from build123d import *

# Parameters (mm, degrees)
F0_R     = 33.1615614797
F1_DEPTH = 79.248
F3_DEPTH = 111.252
F4_T     = -2.54


with BuildPart() as f1:
    # F0 (on Front) → F1 (new body)
    with BuildSketch(Plane.XZ):
        Circle(F0_R)
    extrude(amount=F1_DEPTH)

    # F2 (on face) → F3 (cut)
    with BuildSketch(Plane.XZ.offset(79.248)):
        Polygon((-9.8989819324, -13.7179617404), (5.2176722472, -3.2694421143), (-0.0481573892, 14.3361204783), (-18.4192732631, 14.7684369255), (-24.507417648, -2.5699394088), align=None)
    extrude(amount=-F3_DEPTH, mode=Mode.SUBTRACT)

    # F4
    f4_openings = [f1.faces().sort_by_distance(p)[0] for p in [
        (-32.223611, -79.248, 0),
    ]]
    offset(amount=F4_T, openings=f4_openings, kind=Kind.INTERSECTION)


solid = f1.part
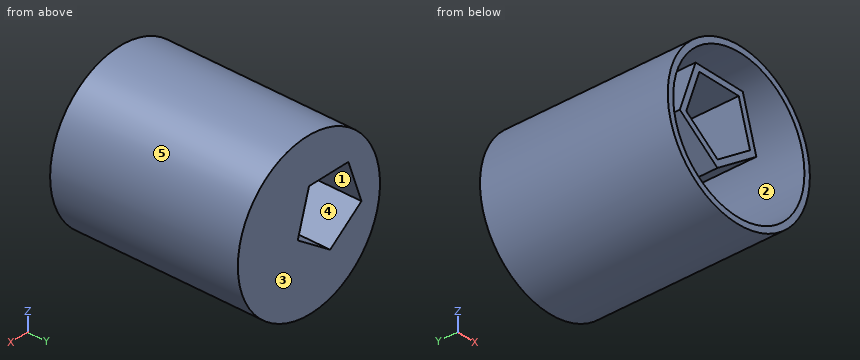
Check sheet for the modelled part. Datum: model origin and axes. Units: mm. Face numbers are marked on the shaded views. A direction names the side the tool comes from. Round coordinates to 2 decimals unless told otherwise and drop trailing zeros. Order: outer loops, then holes, each group sorted by start corner. A loop starts at its lowest first (then second) coordinate and runs counter-clockwise, first axis right, second up.
Q1. Scan lines: L1, parallel to X at y = -51, z = 13; L2, parallel to X at y = -29, z = -6; L3, parallel to Z at x = -2.5, y = -23. Record each from-to range of solid material in increasing order.
Filled sheet:
L1: x = -30.51 to -27.73, -21.73 to -19.04, 0.35 to 3, 27.73 to 30.51
L2: x = -32.61 to -30.03, -24.2 to -20.01, 1.27 to 5.73, 30.03 to 32.61
L3: z = -33.07 to -30.52, -11.69 to -8.6, 14.39 to 16.93, 30.52 to 33.07
Q2. Set-up check for the marked faces 1 and 2: record each of +Z, -Z, +X, -X, +Y, -Y from which the full face is reachable in a straight line by a thin tool's end or side.
Filled sheet:
face 1: +Y, -Y
face 2: -Y
Q3. Cross-section at C-C, the plane x = -6. Enter the section's corners in (y, z), plus the area to 3 significant figures.
Filled sheet:
outline: (-79.25, -32.61) - (0, -32.61) - (0, -11.02) - (-79.25, -11.02) - (-79.25, -14.11) - (-2.54, -14.11) - (-2.54, -30.03) - (-79.25, -30.03) - close; (-79.25, 14.48) - (0, 14.48) - (0, 32.61) - (-79.25, 32.61) - (-79.25, 30.03) - (-2.54, 30.03) - (-2.54, 17.02) - (-79.25, 17.02) - close
area: 929 mm2
Q4. Cross-section at B-B, the plane z = 10. Enter the section's corners in (x, y).
Filled sheet:
outline: (-31.62, -79.25) - (-28.94, -79.25) - (-28.94, -2.54) - (-22.79, -2.54) - (-22.79, -79.25) - (-20.09, -79.25) - (-20.09, 0) - (-31.62, 0) - close; (1.25, -79.25) - (3.9, -79.25) - (3.9, -2.54) - (28.94, -2.54) - (28.94, -79.25) - (31.62, -79.25) - (31.62, 0) - (1.25, 0) - close
Q5. Draft check along X on the marked faces 3, 4 and 5. Enter one of: pulls with the +X half, pulls with the -X half, needs draft (parallel to the pull), parting line crosses it, or undercut.
Filled sheet:
face 3: needs draft
face 4: undercut
face 5: parting line crosses it
Q6. Cross-section at A-A, the plane y = -28.5. Enter the section's corners in (x, z).
Filled sheet:
outline: circle Ø66.32 at (0, 0); (-27.52, -3.47) - (-9.97, -16.86) - (8.18, -4.31) - (1.86, 16.83) - (-20.2, 17.35) - close; hole circle Ø61.24 at (0, 0); hole (-24.51, -2.57) - (-9.9, -13.72) - (5.22, -3.27) - (-0.05, 14.34) - (-18.42, 14.77) - close
Q7. Cross-section at D-D, the plane x = 22.5. Enter the section's corners in (y, z).
Filled sheet:
outline: (-79.25, -24.36) - (0, -24.36) - (0, 24.36) - (-79.25, 24.36) - (-79.25, 20.77) - (-2.54, 20.77) - (-2.54, -20.77) - (-79.25, -20.77) - close
Q8. Depth check by flat-ended pin: P1, Ø10, axis at x = -4.5, y = -61.5, coming from the +Z side; P2, Ø1.5, axis at y = -15, z = -17.5, coming from the -X side; P3, Ø1.5, axis at y = -26, z = 26.5, coming from the -X side. Enter the tip coordinate at first touch or a pass-through.
Filled sheet:
P1: stops at z = 33.16
P2: stops at x = -28.62
P3: stops at x = -20.9
